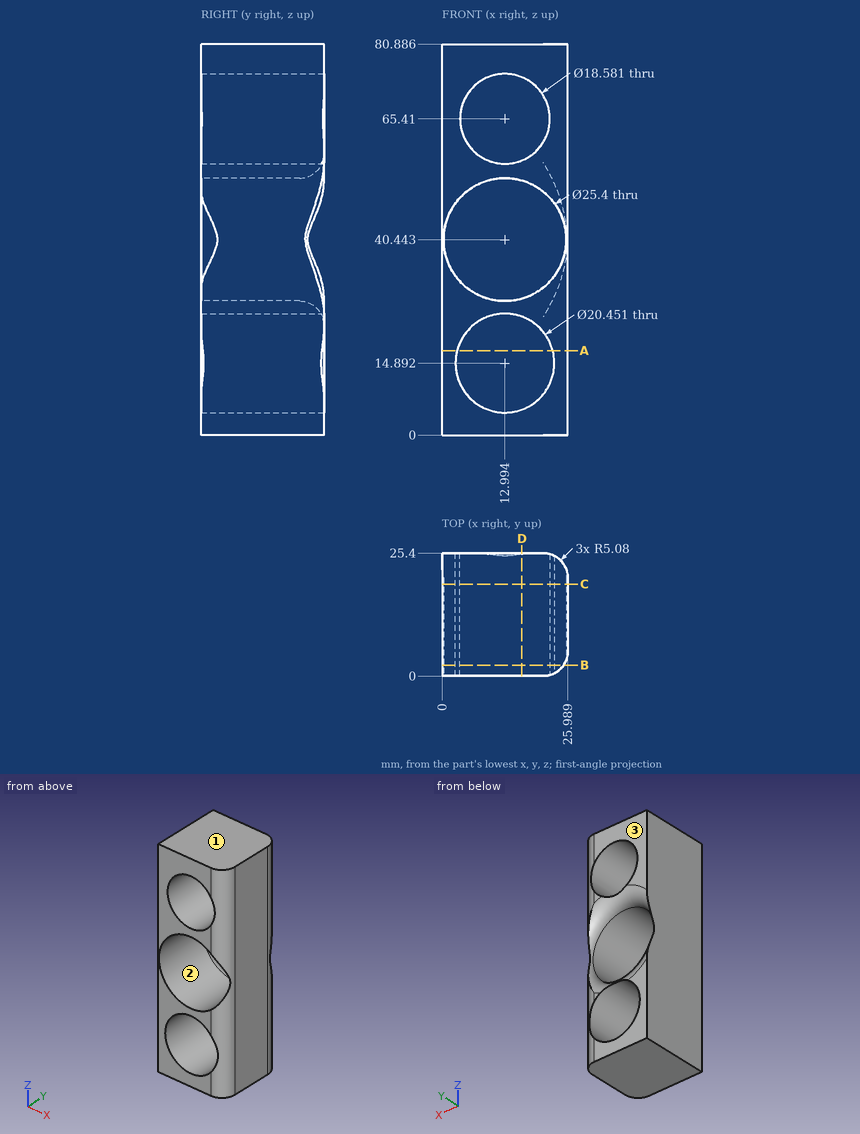
Could you check a few things on this drawing? It's one solid part, dimensions in mm from its lowest x, y, z. Coordinates: 2 decimals unless noted, no trailing zeros. Order: outer loops, then holes, each group sorted by start corner. A loop starts at its lowest first (then second) coordinate and runs counter-clockwise, first axis right, second up. Notation, with made-up numbers: (32, 19.5) - (82, 19.5) arc R23 cw to (82, 54.5) - close; hole circle Ø10 at (40, -17.5). An arc over 180 degrees is marked (long way). Answer as a JSON object with one key per item and string values. Group by question number.
Q1. Imagine slicing it at C-C (y = 19). Please give me the cut outline in (x, z) (1 decimal).
Q2. Imagine slicing it at B-B (y = 2.25). Please give me the cut outline in (x, z) (1 decimal).
Q3. I need wall thicknesses on line 1 (Z direction, x = 7, y = 18) (1 decimal); line 2 (Z direction, x = 7.75, y = 20.75) (1 decimal); line 3 (X direction, y = 15.5, z = 49.5) (1 decimal). Which ranges of each line are inside material? Lowest first, please. Write a range as from..to.
Q4. Will this pin go through, and if not, where does the flat tip stop? P1, Ø4, axis at x = 7.5, z = 60, coming from the -Y side.
Q5. Imagine slicing it at D-D (x = 16.5). Give the number of separate pieces and of enclosed holes in the cut face, and give its area (3 significant figures).
Q6. We'd pull the mould along Z, two halves only. Please class the marked faces 1, 2 and 3: +Z half, -Z half, draft (parallel to the pull), parting line (faces both ways), or undercut.
Q7. Imagine slicing it at A-A (z = 17.5). Please give me the cut outline in (x, y), and give its area (3 significant figures).
Determined:
{
 "1": {"outline": "(0, 0) - (26, 0) - (26, 80.9) - (0, 80.9) - close; hole circle Ø25.4 at (13, 40.4); hole circle Ø20.5 at (13, 14.9); hole circle Ø18.6 at (13, 65.4)"},
 "2": {"outline": "(0, 0) - (25.1, 0) - (25.1, 36.7) arc R12.7 cw (long way) to (25.1, 44.2) - (25.1, 80.9) - (0, 80.9) - close; hole circle Ø20.5 at (13, 14.9); hole circle Ø18.6 at (13, 65.4)"},
 "3": {"line 1": "z = 0..6.6, 23.2..29.2, 51.6..58.3, 72.5..80.9", "line 2": "z = 0..6.1, 23.7..28.9, 52..57.7, 73.1..80.9", "line 3": "x = 0..4.1, 21.9..26"},
 "4": {"P1": "stops at y = 0"},
 "5": {"separate pieces": "4", "enclosed holes": "0", "area": "498 mm2"},
 "6": {"face 1": "+Z half", "face 2": "undercut", "face 3": "draft"},
 "7": {"outline": "(0, 0) - (3.11, 0) - (3.11, 25.4) - (0, 25.4) - close; (22.88, 0.4) arc R5.08 ccw to (25.99, 5.08) - (25.99, 20.32) arc R5.08 ccw to (22.88, 25) - close", "area": "147 mm2"}
}
